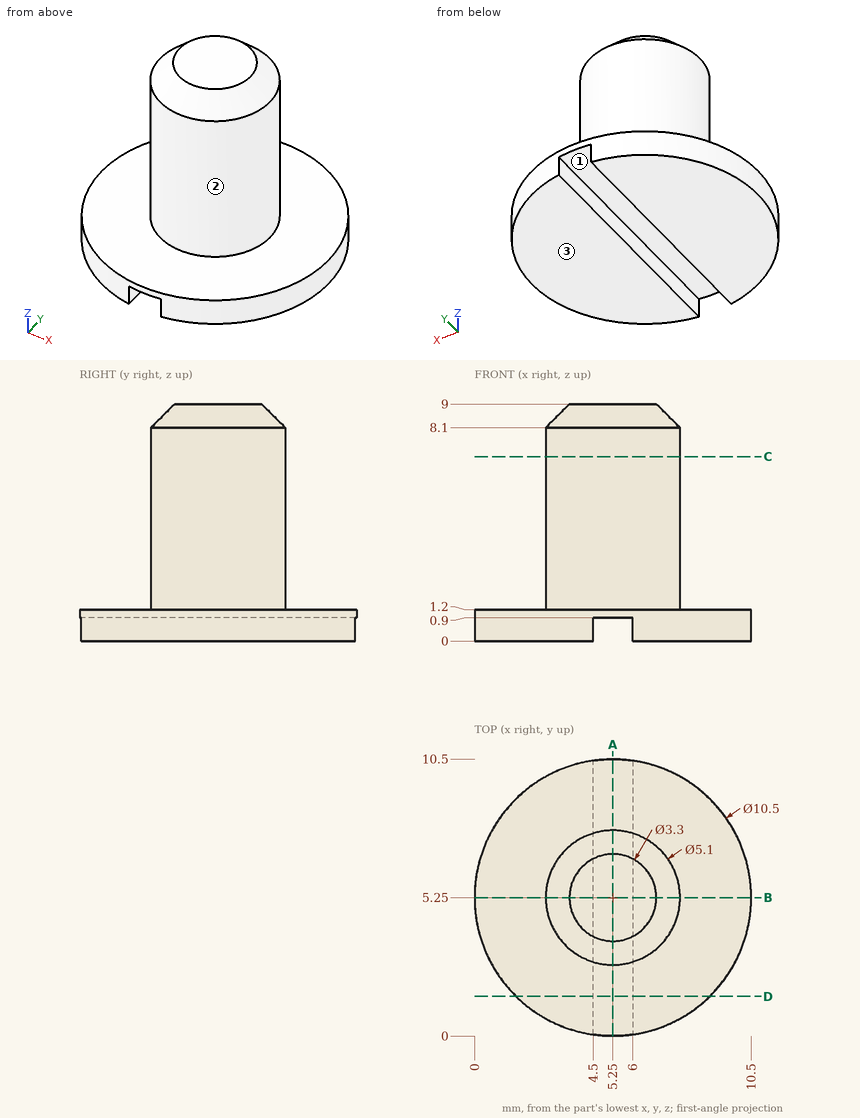
Source: three-view drawing plus pictorial views. Frame: mm from the lowest corner of the part. A direction names the side the tool comes from. Coordinates: 2 decimals unless noted, no trailing zeros. Order: outer loops, then holes, each group sorted by start corner. A loop starts at its lowest first (then second) coordinate and runs counter-clockwise, first axis right, second up. Notation, with made-up numbers: M -6.5,22.25 L 45.5,22.25 A17 ccw 45.5,44.25 Z; hole C 77,61.25 d2. An arc over 180 degrees is marked long. One line per question, with ' | ' between items.
Item 1: Pin query (flat end, axial travel): pin 1 (4 mm diameter, centred on x = 6, z = 7, fed in from -Y); pin 2 (3 mm diameter, centred on y = 9, z = 3, fed in from -X); pin 3 (0.7 mm diameter, centred on y = 4, z = 0.5, fed in from +X). Return the tip coordinate at first contact, or that it passes through.
Geometry results:
pin 1: stops at y = 2.7 | pin 2: stops at x = 4.05 | pin 3: stops at x = 10.42
Item 2: Section C-C (z = 7). Output: boundary loops of the cut face in (x, y), then the cut area to 3 significant figures.
Geometry results:
outline: C 5.25,5.25 d5.1 | area: 20.4 mm^2
Item 3: Section D-D (y = 1.5). Output: boundary loops of the cut face in (x, z).
Geometry results:
outline: M 1.58,0 L 4.5,0 L 4.5,0.9 L 6,0.9 L 6,0 L 8.92,0 L 8.92,1.2 L 1.58,1.2 Z
Item 4: Ray query, line 1 along Z through (x, y) = (6.5, 8); line 2 along Y through (x, z) = (4.5, 7); line 3 along Z through (x, y) = (5.25, 9.5). Return the intervals inside material, ascending.
Geometry results:
line 1: z = 0 to 1.2 | line 2: y = 2.81 to 7.69 | line 3: z = 0.9 to 1.2
Item 5: Section B-B (y = 5.25). Output: boundary loops of the cut face in (x, z), then the cut area to 3 significant figures.
Geometry results:
outline: M 0,0 L 4.5,0 L 4.5,0.9 L 6,0.9 L 6,0 L 10.5,0 L 10.5,1.2 L 7.8,1.2 L 7.8,8.1 L 6.9,9 L 3.6,9 L 2.7,8.1 L 2.7,1.2 L 0,1.2 Z | area: 50.2 mm^2
Item 6: Section A-A (x = 5.25). Output: boundary loops of the cut face in (y, z).
Geometry results:
outline: M 0,0.9 L 10.5,0.9 L 10.5,1.2 L 7.8,1.2 L 7.8,8.1 L 6.9,9 L 3.6,9 L 2.7,8.1 L 2.7,1.2 L 0,1.2 Z
Item 7: Reachability of the marked faces 1, 2 and 3 from +Z, -Z, +X, -X, +Y, -Y: full face, straight path, thin tool, end or side. Return the list, or none.
Geometry results:
face 1: -Z, +Y, -Y | face 2: +Z | face 3: -Z, +X, -X, +Y, -Y
